from build123d import *

# Parameters (mm, degrees)
EXTRUDE_1_DEPTH             = 60
SKETCH_2_R                  = 2
EXTRUDE_2_DEPTH             = 6
SKETCH_3_R                  = 2
SKETCH_3_R_2                = 1.6
CUT_EXTRUDE_3_DEPTH         = 0.5
CHAMFER_1_SIZE              = 0.4
HOLE_WIZARD_M31_D           = 3.2
HOLE_WIZARD_M31_DEPTH       = 10
HOLE_WIZARD_M31_CSINK_D     = 4
HOLE_WIZARD_M31_CSINK_ANGLE = 90
HOLE_WIZARD_M31_TIP         = 0.96137699


with BuildPart() as part:
    # Эскиз1 → Вытянуть1 (new body)
    with BuildSketch(Plane.XY):
        Polygon((0, 4.041451884), (-3.5, 2.020725942), (-3.5, -2.020725942), (0, -4.041451884), (3.5, -2.020725942), (3.5, 2.020725942), align=None)
    extrude(amount=EXTRUDE_1_DEPTH)

    # Эскиз2 → Вытянуть2 (add)
    with BuildSketch(Plane.XY.offset(60)):
        Circle(SKETCH_2_R)
    extrude(amount=EXTRUDE_2_DEPTH)

    # Эскиз3 → Вырез-Вытянуть3 (cut)
    with BuildSketch(Plane.XY.offset(60)):
        Circle(SKETCH_3_R)
        Circle(SKETCH_3_R_2, mode=Mode.SUBTRACT)
    extrude(amount=CUT_EXTRUDE_3_DEPTH, mode=Mode.SUBTRACT)

    # Фаска1
    chamfer_1_edges = [part.edges().sort_by_distance(p)[0] for p in [
        (-2, 0, 66),
        (-2, 0, 60.5),
    ]]
    chamfer(chamfer_1_edges, length=CHAMFER_1_SIZE - 0.0001)  # a hair under: the kernel refuses the full size

    # Отверстие с зазором M31
    with Locations(Plane(origin=(0, 0, 0), x_dir=(-1, 0, 0), z_dir=(0, 0, -1))):
        with Locations((0, 0)):
            CounterSinkHole(HOLE_WIZARD_M31_D / 2, HOLE_WIZARD_M31_CSINK_D / 2, depth=HOLE_WIZARD_M31_DEPTH, counter_sink_angle=HOLE_WIZARD_M31_CSINK_ANGLE)
            with Locations((0, 0, -(HOLE_WIZARD_M31_DEPTH + HOLE_WIZARD_M31_TIP / 2))):  # 118° drill point
                Cone(0, HOLE_WIZARD_M31_D / 2, HOLE_WIZARD_M31_TIP, mode=Mode.SUBTRACT)


solid = part.part
For this review, take the finished solid that the model builds, in its own axes (mm). A direction names the side the tool comes from. Round coordinates to 2 decimals unless told otherwise and drop trailing zeros. Order: outer loops, then holes, each group sorted by start corner. A loop starts at its lowest first (then second) coordinate and runs counter-clockwise, first axis right, second up. Notation, with made-up numbers: M -21,-0.75 L 37,-0.75 A34 ccw 37,33.25 Z; hole C -38,-33 d11. An arc over 180 degrees is marked long. Use a Markdown table: item, result. Add a question column.
Item 1: Insertion check: pin 1 (3.5 mm diameter, centred on x = 0, y = 0, fed in from -Z); pin 2 (1.6 mm diameter, centred on x = 0.5, y = -0.5, fed in from -Z); pin 3 (2 mm diameter, centred on x = 2.5, z = 40, fed in from -Y). Each pin has a flat end and moves straight along its axis. Give the tip position at first contact, or say it passes through.
Item 2: Add section B-B, the plane z = 62. Give the boundary of the cut face in (x, y), then the cut area to 3 significant figures.
Item 3: Mouldability with a two-part tool opening along X and no side actions: class faces 1 (the cylindrical face through (-1.27, -0.97, 5.27)), 2 (the conical face through (0.278, 0.012, 10.794)), 3 (the flat face through (-1.8, -3, 29.6)), 4 (the flat face through (0, 0, 66)) as released by +X, released by -X, zero draft, split by the parting line, or undercut.
Item 4: Add section A-A, the plane z = 15. Give the boundary of the cut face in (x, y).
Item 5: Tool access review of faces 5 (the flat face through (-2, 0, 60)), 6 (the flat face through (-3.5, 0, 30)), 7 (the cylindrical face through (0, -2, 63)): name each direction out of +Z, -Z, +X, -X, +Y, -Y from which nothing blocks a thin tool from reaching the whole face with its end or side.
Item 6: To check wall thickness, follow line 1 along X through (y, z) = (0, 3.5); line 2 along Y through (x, z) = (0, 3.75); line 3 along Z through (x, y) = (0, -3). State the ranges of each line that lie inside material, in increasing order.
Geometry results:
| question | item | result |
|---|---|---|
| 1 | pin 1 | stops at z = 0.25 |
| 1 | pin 2 | stops at z = 10.06 |
| 1 | pin 3 | stops at y = -3.18 |
| 2 | outline | C 0,0 d4 |
| 2 | area | 12.6 mm² |
| 3 | face 1 | undercut |
| 3 | face 2 | undercut |
| 3 | face 3 | released by -X |
| 3 | face 4 | zero draft |
| 4 | outline | M -3.5,-2.02 L 0,-4.04 L 3.5,-2.02 L 3.5,2.02 L 0,4.04 L -3.5,2.02 Z |
| 5 | face 5 | none |
| 5 | face 6 | +Z, -Z, -X, +Y, -Y |
| 5 | face 7 | +Z |
| 6 | line 1 | x = -3.5 to -1.6, 1.6 to 3.5 |
| 6 | line 2 | y = -4.04 to -1.6, 1.6 to 4.04 |
| 6 | line 3 | z = 0 to 60 |
